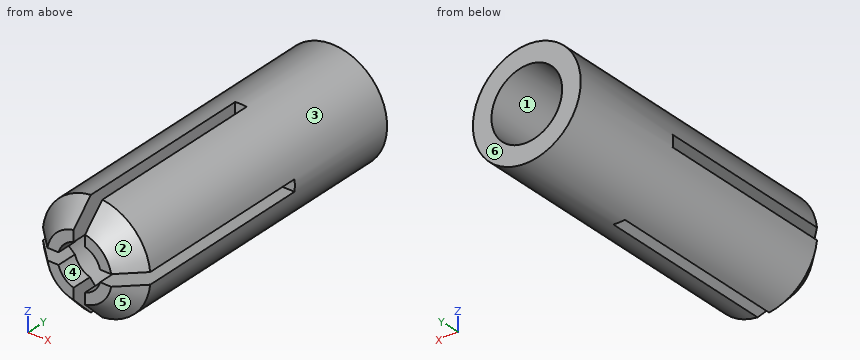
Autodesk Inventor part; units mm, degrees
ref_plane "YZ Plane" through (0, 0, 0) normal (1, 0, 0) x (0, 1, 0)
ref_plane "XZ Plane" through (0, 0, 0) normal (0, 1, 0) x (-1, 0, 0)
ref_plane "XY Plane" through (0, 0, 0) normal (0, 0, 1) x (1, 0, 0)
sketch "Sketch1" plane through (0, 0, 0) normal (0, 1, 0) x (-1, 0, 0)
  circle A0 centre (0, 0) radius 3.75
  dimension "d0" = 7.5
extrude "Extrusion1" add sketch "Sketch1" along normal blind 22
sketch "Sketch2" plane through (0, 22, 0) normal (0, 1, 0) x (1, 0, 0)
  circle A0 centre (0, 0) radius 3.75
hole "Hole1" at (0, 22, 0) direction (0, -1, 0) diameter 4.917 depth 20 tip angle 118
chamfer "Chamfer1" distance 1.5 angle 45 1 edges at (3.75, 0, 0)
sketch "Sketch4" plane through (0, 0, 0) normal (1, 0, 0) x (0, 1, 0)
  line L0 (0, -2.25) -> (0, 2.25)
  line L1 (0, -0.4) -> (14, -0.4)
  line L2 (14, -0.4) -> (14, 0.4)
  line L3 (14, 0.4) -> (0, 0.4)
  line L4 (0, 0.4) -> (0, -0.4)
  point P0 (0, 0)
  point P1 (0, 0.4)
  dimension "d19" = 0.8
  dimension "d20" = 0.4
  dimension "d21" = 14
sketch "Sketch5" plane through (0, 0, 0) normal (0, -1, 0) x (1, 0, 0)
  circle A0 centre (0, 0) radius 1.5
  dimension "d16" = 3
extrude "Extrusion3" cut sketch "Sketch5" against normal through all
extrude "Extrusion4" cut sketch "Sketch4" along normal through all both and the other way through all
pattern_circular "Circular Pattern1" count 4 over 360 about axis through (0, 0, 0) along (0, 1, 0) of "Extrusion4"
properties part number "clamping_insert"
The listing builds one solid part. Answer for the finished solid, in the listing's coordinates (mm). Face numbers are marked on the shaded views. A direction names the side the tool comes from. Give positions to 0.01 mm unless a question says otherwise; leave off trailing zeros. Write each loop counter-clockwise with the first axis right and the second up, starting at its lowest first coordinate (ties: lowest second). Pieces come first, ordered by that corner, then holes. Notation, with made-up numbers: (-8.75, 54) -> (18.25, 54) arc R18 cw to (18.25, 77) -> close; hole circle Ø6 at (-16, 9). An arc over 180 degrees is marked (long way). Write item = value, one per line. Start each with the question number.
1) The part is cut by section D-D, the plane y = 17.25. Determine the outline of the cut face in (x, z).
2) The part is cut by section B-B, the plane x = 0. Determine the outline of the cut face in (y, z).
3) Straight lines are drawn through the part: line 1 along X through (y, z) = (14.75, 0); line 2 along Z through (x, y) = (-0.75, 21); line 3 along Z through (x, y) = (-1.75, 8). For each, find the intervals that lie inside material, in ascending order.
4) Determine the mould class of the marked faces 3, 4, 5 and 6 for opening direction X: +X half, -X half, draft (parallel to the pull), parting line (faces both ways), or undercut.
5) The part is cut by section A-A, the plane y = 4.5. Determine the outline of the cut face in (x, z), and give its area (3 significant figures).
6) The part is cut by section C-C, the plane z = 0. Determine the outline of the cut face in (x, y), and give its area (3 significant figures).
7) Which of the six approach directions +Z, -Z, +X, -X, +Y, -Y give full straight-line access (tool end or side, diameter ignored) to the marked faces 1 and 2?
8) Each of these flat-tipped pins is pushed along its axis until it touches: pin 1 (0.7 mm diameter, centred on y = 5, z = 3, fed in from -X); pin 2 (0.7 mm diameter, centred on y = 3.5, z = -2, fed in from +X); pin 3 (1.8 mm diameter, centred on x = -3, y = 9.5, fed in from -Z). Where does it stop, or does it pass through?
Solutions:
q1.outline = circle Ø7.5 at (0, 0); hole circle Ø4.92 at (0, 0)
q2.outline = (14, -3.75) -> (22, -3.75) -> (22, -2.46) -> (14, -2.46) -> close; (14, 2.46) -> (22, 2.46) -> (22, 3.75) -> (14, 3.75) -> close
q3.line_1 = -3.75 to -2.46, 2.46 to 3.75
q3.line_2 = -3.67 to -2.34, 2.34 to 3.67
q3.line_3 = -3.32 to -1.73, 1.73 to 3.32
q4.face_3 = parting line
q4.face_4 = undercut
q4.face_5 = +X half
q4.face_6 = draft
q5.outline = (-3.73, -0.4) arc R3.75 ccw to (-0.4, -3.73) -> (-0.4, -2.43) arc R2.46 cw to (-2.43, -0.4) -> close; (-3.73, 0.4) -> (-2.43, 0.4) arc R2.46 cw to (-0.4, 2.43) -> (-0.4, 3.73) arc R3.75 ccw to start; (0.4, -3.73) arc R3.75 ccw to (3.73, -0.4) -> (2.43, -0.4) arc R2.46 cw to (0.4, -2.43) -> close; (0.4, 2.43) arc R2.46 cw to (2.43, 0.4) -> (3.73, 0.4) arc R3.75 ccw to (0.4, 3.73) -> close
q5.area = 21.0 mm²
q6.outline = (-3.75, 14) -> (-2.46, 14) -> (-2.46, 22) -> (-3.75, 22) -> close; (2.46, 14) -> (3.75, 14) -> (3.75, 22) -> (2.46, 22) -> close
q6.area = 20.7 mm²
q7.face_1 = +Y
q7.face_2 = +Z, +X, -Y
q8.pin_1 = -2.65
q8.pin_2 = 3.37
q8.pin_3 = -3.11
